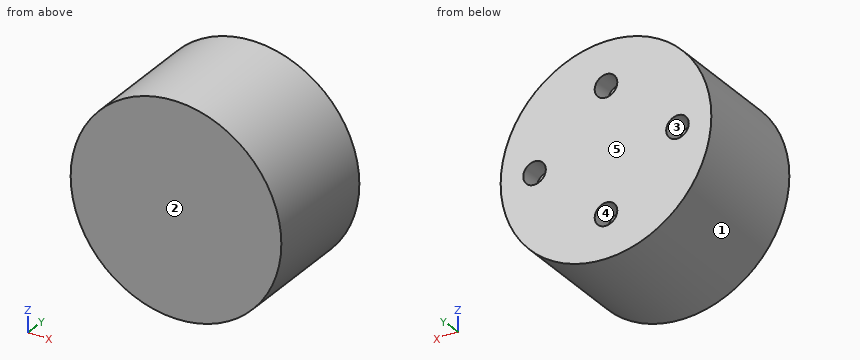
from build123d import *

# Parameters (mm, degrees)
F0_R     = 14
F1_DEPTH = 8
F2_R     = 1.5
F3_DEPTH = 2.8


with BuildPart() as f1:
    # F0 (on Front) → F1 (new body, symmetric)
    with BuildSketch(Plane.XZ):
        Circle(F0_R)
    extrude(amount=F1_DEPTH, both=True)

    # F2 (on face) → F3 (cut)
    with BuildSketch(Plane(origin=(0, 8, 0), x_dir=(-1, 0, 0), z_dir=(0, 1, 0))):
        with Locations((0, 8.25)):
            Circle(F2_R)
        with Locations((0, -8.25)):
            Circle(F2_R)
        with Locations((9.5, 0)):
            Circle(F2_R)
        with Locations((-9.5, 0)):
            Circle(F2_R)
    extrude(amount=-F3_DEPTH, mode=Mode.SUBTRACT)


solid = f1.part
Here's how the part is built. I have some questions about the finished solid (model axes, mm). Face numbers are marked on the shaded views. A direction names the side the tool comes from. Round coordinates to 2 decimals unless told otherwise and drop trailing zeros. Order: outer loops, then holes, each group sorted by start corner. A loop starts at its lowest first (then second) coordinate and runs counter-clockwise, first axis right, second up. Notation, with made-up numbers: M 86.5,44 L 97.5,44 A16 cw 97.5,53 Z; hole C -40,62 d1. An arc over 180 degrees is marked long. One line per question, with ' | ' between items.
1) I'm going to push flat-ended pins straight in: pin 1 Ø6 at (y, z) = (-3, -4.5) entering from -X; pin 2 Ø3 at (x, y) = (-3.5, 0) entering from +Z; pin 3 Ø1.8 at (x, z) = (0, 8.25) entering from +Y. Where does each tip first touch, or does it pass through?
Checked values:
pin 1: stops at x = -13.92 | pin 2: stops at z = 13.86 | pin 3: stops at y = 5.2
2) On a 3-axis mill with a long thin cutter (end or side, diameter ignored), from which of +Z, -Z, +X, -X, +Y, -Y can I reach the whole of each face in a straight line? I mean the marked faces 4 and 5. Say none if no direction works.
Checked values:
face 4: +Y | face 5: +Z, -Z, +X, -X, +Y
3) I need wall thicknesses on line 1 (Z direction, x = 0, y = 5.9); line 2 (Z direction, x = 9.5, y = 7.25); line 3 (X direction, y = 6.25, z = 6). Which ranges of each line are inside material? Lowest first, please.
Checked values:
line 1: z = -14 to -9.75, -6.75 to 6.75, 9.75 to 14 | line 2: z = -10.28 to -1.5, 1.5 to 10.28 | line 3: x = -12.65 to 12.65
4) Imagine slicing it at B-B, the plane z = 0. Write out the boundary of the cut face in (x, y).
Checked values:
outline: M -14,-8 L 14,-8 L 14,8 L 11,8 L 11,5.2 L 8,5.2 L 8,8 L -8,8 L -8,5.2 L -11,5.2 L -11,8 L -14,8 Z
5) Imagine slicing it at C-C, the plane y = 3.5. Write out the boundary of the cut face in (x, z), plus the area to 3 significant figures.
Checked values:
outline: C 0,0 d28 | area: 616 mm²
6) Imagine slicing it at D-D, the plane x = 9.5. Write out the boundary of the cut face in (y, z).
Checked values:
outline: M -8,-10.28 L 8,-10.28 L 8,-1.5 L 5.2,-1.5 L 5.2,1.5 L 8,1.5 L 8,10.28 L -8,10.28 Z
7) Imagine slicing it at A-A, the plane x = 0. Write out the boundary of the cut face in (y, z), plus the area to 3 significant figures.
Checked values:
outline: M -8,-14 L 8,-14 L 8,-9.75 L 5.2,-9.75 L 5.2,-6.75 L 8,-6.75 L 8,6.75 L 5.2,6.75 L 5.2,9.75 L 8,9.75 L 8,14 L -8,14 Z | area: 431 mm²
8) We'd pull the mould along Z, two halves only. Please class the marked faces 1, 2 and 3: released by +Z, released by -Z, zero draft, split by the parting line, or undercut.
Checked values:
face 1: split by the parting line | face 2: zero draft | face 3: undercut
